Check sheet for the drawn part. Datum: minimum x, y, z corner. Units: mm. Coordinates: 2 decimals unless noted, no trailing zeros. Order: outer loops, then holes, each group sorted by start corner. A loop starts at its lowest first (then second) coordinate and runs counter-clockwise, first axis right, second up. Notation, with made-up numbers: (87, 9.5) - (123, 9.5) arc R22 ccw to (123, 39.5) - close; hole circle Ø4 at (82, -5). An arc over 180 degrees is marked (long way). Answer as CSV lines item,"result". Start each with the question number.
1. Material ranges on L1, parallel to Z at x = 29, y = 2.15; L2, parallel to Y at x = 31, z = 1.4; L3, parallel to Y at x = 15.5, z = 0.4, recorded low to high. Write a range as [from, to].
2. Go/stop test with a flat-tipped pin: pin 1 (1.5 mm diameter, centred on x = 15, y = 2.5, fed in from +Z). Record where the tip stops, or that it passes through.
3. Section check A-A (x = 11). Record the cut outline in (y, z), and give its area (3 significant figures).
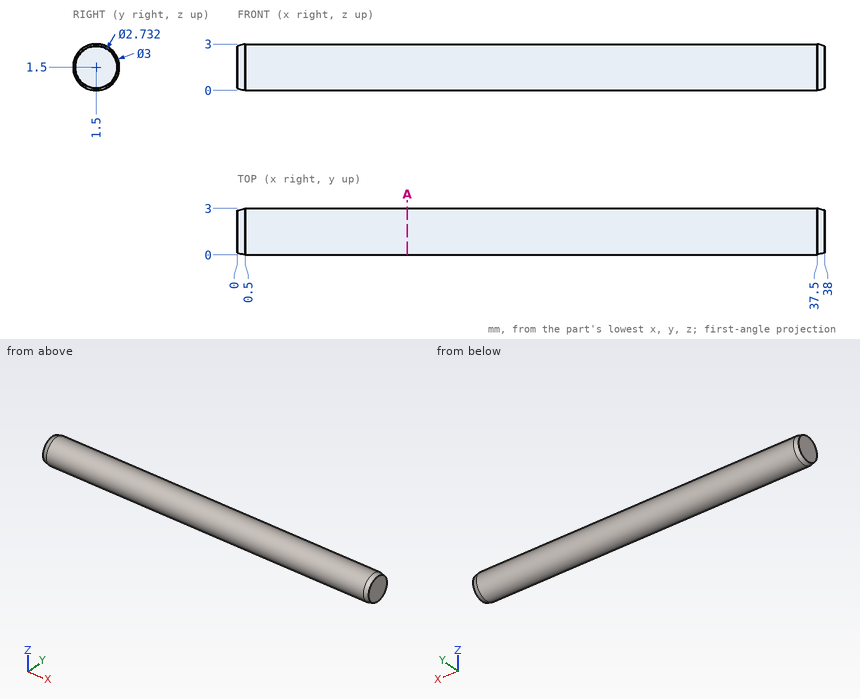
Evaluation:
1,L1,"z = [0.15, 2.85]"
1,L2,"y = [0, 3]"
1,L3,"y = [0.48, 2.52]"
2,pin 1,"stops at z = 2.98"
3,outline,"circle Ø3 at (1.5, 1.5)"
3,area,"7.07 mm²"
